```python
from build123d import *

# Parameters (mm, degrees)
SKETCH_1_W      = 40
SKETCH_1_H      = 35
SKETCH_1_R      = 2.7
EXTRUDE_1_DEPTH = 3.5
SKETCH_2_W      = 40
SKETCH_2_H      = 4
EXTRUDE_2_DEPTH = 7


with BuildPart() as part:
    # 草图1 → 凸台-拉伸1 (new, symmetric)
    with BuildSketch(Plane.XY):
        with Locations((0, 17.5)):
            Rectangle(SKETCH_1_W, SKETCH_1_H)
        with Locations((6, 22)):
            Circle(SKETCH_1_R, mode=Mode.SUBTRACT)
    extrude(amount=EXTRUDE_1_DEPTH, both=True)

    # 草图2 → 凸台-拉伸2 (add)
    with BuildSketch(Plane.XY):
        with Locations((0, 2)):
            Rectangle(SKETCH_2_W, SKETCH_2_H)
    extrude(amount=EXTRUDE_2_DEPTH)


solid = part.part
```
Read the model definition and answer for the solid it produces. Units are mm, in the model's axes. A direction names the side the tool comes from. Give positions to 0.01 mm unless a question says otherwise; leave off trailing zeros. Order: outer loops, then holes, each group sorted by start corner. A loop starts at its lowest first (then second) coordinate and runs counter-clockwise, first axis right, second up. Notation, with made-up numbers: (75, -38.5) -> (108, -38.5) arc R26 cw to (108, -22.5) -> close; hole circle Ø1 at (53.25, -1). An arc over 180 degrees is marked (long way). Write item = value, one per line.
1. A cutting plane is placed at D-D, the plane x = 13.5. Write down the section's boundary in (y, z), and give its area (3 significant figures).
Numbers:
outline = (0, -3.5) -> (35, -3.5) -> (35, 3.5) -> (4, 3.5) -> (4, 7) -> (0, 7) -> close
area = 259 mm²
2. For faces 4 (the face through (0, 4, 5)), 5 (the face through (0, 18, -3.5)), determine the directions among +Z, -Z, +X, -X, +Y, -Y from which every point of the face is accessible in a straight line to the end or side of a thin tool.
Numbers:
face_4 = +Z, +X, -X, +Y
face_5 = -Z, +X, -X, +Y, -Y
3. A cutting plane is placed at A-A, the plane x = 6. Write down the section's boundary in (y, z), and give its area (3 significant figures).
Numbers:
outline = (0, -3.5) -> (19.3, -3.5) -> (19.3, 3.5) -> (4, 3.5) -> (4, 7) -> (0, 7) -> close; (24.7, -3.5) -> (35, -3.5) -> (35, 3.5) -> (24.7, 3.5) -> close
area = 221 mm²
4. Given pin 1 (4 mm diameter, centred on x = 14.5, z = 3.5, fed in from -Y); pin 2 (3 mm diameter, centred on x = -7.5, y = 10.5, fed in from +Z), each flat-ended and moving along its own axis, determine where each tip first touches the part or whether it passes through.
Numbers:
pin_1 = 0
pin_2 = 3.5
5. A cutting plane is placed at B-B, the plane y = 22. Write down the section's boundary in (x, z).
Numbers:
outline = (-20, -3.5) -> (3.3, -3.5) -> (3.3, 3.5) -> (-20, 3.5) -> close; (8.7, -3.5) -> (20, -3.5) -> (20, 3.5) -> (8.7, 3.5) -> close
6. The mould has two halves that part along Y. Classify faces 1 (the face through (0, 2, 7)), 2 (the face through (5.649, 24.677, -0.049)), 3 (the face through (0, 0, 2)): +Y half, -Y half, draft (parallel to the pull), parting line (faces both ways), or undercut.
Numbers:
face_1 = draft
face_2 = undercut
face_3 = -Y half
7. A cutting plane is placed at C-C, the plane z = 2.75. Write down the section's boundary in (x, y), and give its area (3 significant figures).
Numbers:
outline = (-20, 0) -> (20, 0) -> (20, 35) -> (-20, 35) -> close; hole circle Ø5.4 at (6, 22)
area = 1,380 mm²
8. Straight lines are drawn through the part: line 1 along Y through (x, z) = (6, -2); line 2 along Z through (x, y) = (11.5, 12.5); line 3 along Y through (x, z) = (6, 6.5). For each, find the intervals that lie inside material, in ascending order.
Numbers:
line_1 = 0 to 19.3, 24.7 to 35
line_2 = -3.5 to 3.5
line_3 = 0 to 4
